The model under review builds one solid part; all positions refer to its coordinate system, in mm. A direction names the side the tool comes from. Round coordinates to 2 decimals unless told otherwise and drop trailing zeros. Loops run counter-clockwise (first coordinate to the right, second up) from the corner with the lowest first, then second, coordinate; pieces in that order, holes last. Notation, with made-up numbers: (-32.5, -35) - (25.5, -35) arc R14 ccw to (25.5, -15) - close; hole circle Ø6 at (3.5, -21). An arc over 180 degrees is marked (long way). Answer as CSV lines item,"result".
from build123d import *

# Parameters (mm, degrees)
SKETCH_1_W          = 40
SKETCH_1_H          = 40
EXTRUDE_1_DEPTH     = 40
SKETCH_2_W          = 34
SKETCH_2_H          = 34
CUT_EXTRUDE_1_DEPTH = 37
FILLET_1_R          = 2


with BuildPart() as part:
    # 草图1 → 凸台-拉伸1 (new body)
    with BuildSketch(Plane(origin=(0, 0, 0), x_dir=(1, 0, 0), z_dir=(0, 1, 0))):
        with Locations((20, -20)):
            Rectangle(SKETCH_1_W, SKETCH_1_H)
    extrude(amount=EXTRUDE_1_DEPTH)

    # 草图2 → 切除-拉伸1 (cut)
    with BuildSketch(Plane(origin=(0, 40, 0), x_dir=(1, 0, 0), z_dir=(0, 1, 0))):
        with Locations((20, -20)):
            Rectangle(SKETCH_2_W, SKETCH_2_H)
    extrude(amount=-CUT_EXTRUDE_1_DEPTH, mode=Mode.SUBTRACT)

    # 圆角1
    fillet_1_edges = [part.edges().sort_by_distance(p)[0] for p in [
        (0, 20, 0),
        (40, 20, 0),
        (40, 20, 40),
        (0, 20, 40),
    ]]
    fillet(fillet_1_edges, radius=FILLET_1_R)


solid = part.part
1. Tool access review of faces 1 (the face through (20, 22, 3)), 2 (the face through (0.57, 20.28, 39.4)): name each direction out of +Z, -Z, +X, -X, +Y, -Y from which nothing blocks a thin tool from reaching the whole face with its end or side.
Numbers:
face 1,"+Y"
face 2,"+Z, -X, +Y, -Y"
2. Take a section at A-A (y = 14). State the section outline as (x, z) points.
Numbers:
outline,"(0, 2) arc R2 ccw to (2, 0) - (38, 0) arc R2 ccw to (40, 2) - (40, 38) arc R2 ccw to (38, 40) - (2, 40) arc R2 ccw to (0, 38) - close; hole (3, 3) - (37, 3) - (37, 37) - (3, 37) - close"
3. Wall thickness on probe 1 along Z at (x, y) = (5.5, 16); probe 2 along Y at (x, z) = (27.5, 35): over which ranges is each line inside the solid? List them lowest first.
Numbers:
probe 1,"z = 0 to 3, 37 to 40"
probe 2,"y = 0 to 3"
4. Take a section at B-B (x = 25). State the section outline as (y, z) points, plus the area to 3 significant figures.
Numbers:
outline,"(0, 0) - (40, 0) - (40, 3) - (3, 3) - (3, 37) - (40, 37) - (40, 40) - (0, 40) - close"
area,"342 mm²"
5. Draft analysis for pull direction Z (two halves, no side actions). For faces 3 (the face through (20, 22, 37)), 4 (the face through (0, 20, 20)), 5 (the face through (39.4, 20.28, 0.57)), state which applies: +Z half, -Z half, draft (parallel to the pull), parting line (faces both ways), or undercut.
Numbers:
face 3,"undercut"
face 4,"draft"
face 5,"-Z half"
6. Take a section at C-C (z = 17). State the section outline as (x, y) points.
Numbers:
outline,"(0, 0) - (40, 0) - (40, 40) - (37, 40) - (37, 3) - (3, 3) - (3, 40) - (0, 40) - close"
